```python
from build123d import *

# Parameters (mm, degrees)
SKETCH1_R                    = 8
BOSS_EXTRUDE1_DEPTH          = 3
SKETCH2_R                    = 1.25
CUT_EXTRUDE1_DEPTH           = 12.704699911
SKETCH3_R                    = 15
BOSS_EXTRUDE2_DEPTH          = 3
CHAMFER1_SIZE                = 5
CHAMFER1_SIZE_2              = 3.004303095
SKETCH4_W                    = 15
SKETCH4_H                    = 2
CUT_EXTRUDE2_DEPTH           = 1.5
CHAMFER2_SIZE                = 0.25
CIRPATTERN1_COUNT            = 8
CHAMFER2_OF_CIRPATTERN1_SIZE = 0.25
FILLET1_R                    = 0.5


with BuildPart() as part:
    # Sketch1 → Boss-Extrude1 (new body)
    with BuildSketch(Plane(origin=(0, 0, 0), x_dir=(1, 0, 0), z_dir=(0, 1, 0))):
        with Locations(Location((0, 0, 0), (0, 0, 270))):
            Circle(SKETCH1_R)
    extrude(amount=BOSS_EXTRUDE1_DEPTH)

    # Sketch2 → Cut-Extrude1 (cut, through all)
    with BuildSketch(Plane(origin=(0, 3, 0), x_dir=(1, 0, 0), z_dir=(0, 1, 0))):
        with Locations(Location((-3.25, 0, 0), (0, 0, 270))):
            Circle(SKETCH2_R)
        with Locations(Location((3.25, 0, 0), (0, 0, 270))):
            Circle(SKETCH2_R)
    extrude(amount=-CUT_EXTRUDE1_DEPTH, mode=Mode.SUBTRACT)

    # Sketch3 → Boss-Extrude2 (add)
    with BuildSketch(Plane.XZ):
        with Locations(Location((0, 0, 0), (0, 0, 270))):
            Circle(SKETCH3_R)
    extrude(amount=BOSS_EXTRUDE2_DEPTH)

    # Chamfer1
    # the kernel refuses this chamfer: 5, 3.004303095 mm, written as the material it adds along each edge
    with BuildSketch(Plane(origin=(0, 0, 0), x_dir=(0, 0, 1), z_dir=(-1, 0, 0))) as chamfer1_piece_1_section:
        Polygon((8 + CHAMFER1_SIZE, 0), (8, CHAMFER1_SIZE_2), (8, 0), align=None)
    chamfer1_piece_1 = revolve(axis=Axis((0, 0, 0), (0, 1, 0)), mode=Mode.PRIVATE)
    chamfer1_piece_1 = split(chamfer1_piece_1, bisect_by=Plane(origin=(0, 3, -10.54798904), z_dir=(0, -1, 0)), keep=Keep.TOP, mode=Mode.PRIVATE)
    add(chamfer1_piece_1)

    # Sketch4 → Cut-Extrude2 (cut)
    with BuildSketch(Plane.XZ.offset(3)):
        with Locations((7.5, 0)):
            Rectangle(SKETCH4_W, SKETCH4_H)
    cut_extrude2 = extrude(amount=-CUT_EXTRUDE2_DEPTH, mode=Mode.SUBTRACT)

    # Chamfer2
    chamfer2_edges = [part.edges().sort_by_distance(p)[0] for p in [
        (7.483314774, -3, 1),
        (7.483314774, -3, -1),
    ]]
    chamfer(chamfer2_edges, length=CHAMFER2_SIZE)

    # CirPattern1: Cut-Extrude2 ×8 about axis
    cirpattern1_axis = Axis((0, 0, 0), (0, 1, 0))
    for i in range(1, CIRPATTERN1_COUNT):
        add(cut_extrude2.rotate(cirpattern1_axis, i * 360 / CIRPATTERN1_COUNT), mode=Mode.SUBTRACT)

    # Chamfer2 of CirPattern1
    chamfer2_of_cirpattern1_edges = [part.edges().sort_by_distance(p)[0] for p in [
        (5.998609403, -3, -4.584395841),
        (4.584395841, -3, -5.998609403),
        (1, -3, -7.483314774),
        (-1, -3, -7.483314774),
        (-4.584395841, -3, -5.998609403),
        (-5.998609403, -3, -4.584395841),
        (-7.483314774, -3, -1),
        (-7.483314774, -3, 1),
        (-5.998609403, -3, 4.584395841),
        (-4.584395841, -3, 5.998609403),
        (-1, -3, 7.483314774),
        (1, -3, 7.483314774),
        (4.584395841, -3, 5.998609403),
        (5.998609403, -3, 4.584395841),
    ]]
    chamfer(chamfer2_of_cirpattern1_edges, length=CHAMFER2_OF_CIRPATTERN1_SIZE)

    # Fillet1
    # the kernel refuses this fillet: 0.5 mm, written as the material it takes off along each edge
    with BuildSketch(Plane(origin=(1, -1.5, -2.414213562), x_dir=(0, 0, -1), z_dir=(0, -1, 0)), Plane(origin=(-1, -1.5, 2.414213562), x_dir=(0, 0, 1), z_dir=(0, -1, 0)), Plane(origin=(1, -1.5, 2.414213562), x_dir=(0.7071067811865474, 0, 0.7071067811865477), z_dir=(0, -1, 0)), Plane(origin=(2.414213562, -1.5, -1), x_dir=(0.7071067811865472, 0, -0.7071067811865478), z_dir=(0, -1, 0))) as fillet1_piece_1:
        with BuildLine():
            CenterArc((FILLET1_R * 2.41421356237, FILLET1_R), FILLET1_R, 135, 135)
            Line((FILLET1_R * 1.70710678119, FILLET1_R * 1.70710678119), (0, 0))
            Line((0, 0), (FILLET1_R * 2.41421356237, 0))
        make_face()
    extrude(amount=4.267766953, mode=Mode.SUBTRACT)
    with BuildSketch(Plane(origin=(-1, -1.5, -2.414213562), x_dir=(0, 0, -1), z_dir=(0, -1, 0)), Plane(origin=(-2.414213562, -1.5, -1), x_dir=(-0.7071067811865478, 0, -0.7071067811865474), z_dir=(0, -1, 0)), Plane(origin=(-2.414213562, -1.5, 1), x_dir=(-1, 0, 0), z_dir=(0, -1, 0)), Plane(origin=(2.414213562, -5.767766953, 1), x_dir=(1, 0, 0), z_dir=(0, 1, 0))) as fillet1_piece_2:
        with BuildLine():
            CenterArc((FILLET1_R * 2.41421356237, -FILLET1_R), FILLET1_R, 90, 135)
            Line((FILLET1_R * 1.70710678119, -FILLET1_R * 1.70710678119), (0, 0))
            Line((0, 0), (FILLET1_R * 2.41421356237, 0))
        make_face()
    extrude(amount=4.267766953, mode=Mode.SUBTRACT)


solid = part.part
```
Work out the finished part from the listing and answer in its coordinate system (mm). A direction names the side the tool comes from. Coordinates: 2 decimals unless noted, no trailing zeros. Loops run counter-clockwise (first coordinate to the right, second up) from the corner with the lowest first, then second, coordinate; pieces in that order, holes last. Notation, with made-up numbers: (32, -32) - (38, -32) arc R21 ccw to (38, -18) - close; hole circle Ø7 at (46.25, -26.75). An arc over 180 degrees is marked (long way). Use a Markdown table: item, result.
Item 1: Find section B-B, the plane z = 0. Determine the outline of the cut face in (x, y), and give its area (3 significant figures).
Evaluation:
| item | result |
|---|---|
| outline | (-15, -1.5) - (15, -1.5) - (15, 0) - (13, 0) - (8.01, 3) - (4.5, 3) - (4.5, 0) - (2, 0) - (2, 3) - (-2, 3) - (-2, 0) - (-4.5, 0) - (-4.5, 3) - (-8.01, 3) - (-13, 0) - (-15, 0) - close |
| area | 93.0 mm2 |
Item 2: Consider probe 1 along X at (y, z) = (-1.75, -1.25); probe 2 along X at (y, z) = (1.75, 0); probe 3 along X at (y, z) = (-2.25, -4). Determine where each line is inside the solid, lowest interval first. Write a range as from..to.
Evaluation:
| item | result |
|---|---|
| probe 1 | x = -14.95..-3.19, 3.19..14.95 |
| probe 2 | x = -10.09..-4.5, -2..2, 4.5..10.09 |
| probe 3 | x = -14.46..-5.41, -2.59..-1, 1..2.59, 5.41..14.46 |
Item 3: Find section A-A, the plane x = 0. Determine the outline of the cut face in (y, z), and give its area (3 significant figures).
Evaluation:
| item | result |
|---|---|
| outline | (-1.5, -15) - (0, -15) - (0, -13) - (3, -8.01) - (3, 8.01) - (0, 13) - (0, 15) - (-1.5, 15) - close |
| area | 108 mm2 |
Item 4: Given pin 1 Ø10 at (x, z) = (9.5, 3.5) entering from +Y; pin 2 Ø0.6 at (x, y) = (-9.5, -2) entering from +Z; pin 3 Ø1.4 at (x, y) = (8.5, -2.5) entering from -Z; pin 4 Ø0.8 at (x, z) = (-3, 0.5) entering from +Y, each flat-ended and moving along its own axis, determine where each tip first touches the part or whether it passes through.
Evaluation:
| item | result |
|---|---|
| pin 1 | stops at y = 3 |
| pin 2 | stops at z = 11.85 |
| pin 3 | stops at z = -12.81 |
| pin 4 | stops at y = 0 |
Item 5: For faces 4 (the flat face through (-7.16, -2.88, -5.56)), 5 (the flat face through (5, -3, -10)), 6 (the flat face through (-3, 0, 0)), 7 (the flat face through (9, -2, -1)), determine the directions among +Z, -Z, +X, -X, +Y, -Y from which every point of the face is accessible in a straight line to the end or side of a thin tool.
Evaluation:
| item | result |
|---|---|
| face 4 | -Y |
| face 5 | +Z, -Z, +X, -X, -Y |
| face 6 | +Y |
| face 7 | +X, -X, -Y |
Item 6: Find section C-C, the plane y = -0.75. Determine the outline of the cut face in (x, z).
Evaluation:
| item | result |
|---|---|
| outline | circle Ø30 at (0, 0) |
Item 7: The mould has two halves that part along Z. Classify faces 1 (the conical face through (-5.02, 2.854, -6.547)), 2 (the cylindrical face through (3.163, -2.261, 1.301)), 3 (the flat face through (1, -2, -9)): +Z half, -Z half, draft (parallel to the pull), parting line (faces both ways), or undercut.
Evaluation:
| item | result |
|---|---|
| face 1 | parting line |
| face 2 | undercut |
| face 3 | draft |
Item 8: Find section D-D, the plane y = 1.75. Determine the outline of the cut face in (x, z).
Evaluation:
| item | result |
|---|---|
| outline | circle Ø20.18 at (0, 0); hole circle Ø2.5 at (-3.25, 0); hole circle Ø2.5 at (3.25, 0) |
